```python
from build123d import *

# Parameters (mm, degrees)
F1_DEPTH = 50
F2_R     = 3.15
F3_DEPTH = 2.5
F4_R     = 3.15
F5_DEPTH = 1
F6_R     = 5


with BuildPart() as f1:
    # F0 (on Top) → F1 (new body)
    with BuildSketch(Plane.XY):
        with BuildLine():
            ThreePointArc((4.9458041958, 3.6553414145), (0, -6.15), (-4.9458041958, 3.6553414145))
            ThreePointArc((-4.9458041958, 3.6553414145), (-4.7531001977, 4.3283874081), (-5.0490024533, 4.9628695557))
            Line((-5.0490024533, 4.9628695557), (-5.7683657215, 5.669960926))
            ThreePointArc((-5.7683657215, 5.669960926), (-6.5394133994, 5.9543407148), (-7.2631501723, 5.5649932232))
            ThreePointArc((-7.2631501723, 5.5649932232), (-8.6851191985, -2.8794451737), (-2.5, -8.8018463972))
            Line((-2.5, -8.8018463972), (2.5, -8.8018463972))
            ThreePointArc((2.5, -8.8018463972), (8.6851191985, -2.8794451737), (7.2631501723, 5.5649932232))
            ThreePointArc((7.2631501723, 5.5649932232), (6.5394133994, 5.9543407148), (5.7683657215, 5.669960926))
            Line((5.7683657215, 5.669960926), (5.0490024533, 4.9628695557))
            ThreePointArc((5.0490024533, 4.9628695557), (4.7531001977, 4.3283874081), (4.9458041958, 3.6553414145))
        make_face()
    extrude(amount=F1_DEPTH)

    # F2 (on Right) → F3 (join, symmetric)
    with BuildSketch(Plane.YZ):
        with BuildLine():
            Line((-41.1023570115, 34.5058199478), (-8.8018463972, 0))
            Line((-8.8018463972, 0), (-8.8018463972, 50))
            Line((-8.8018463972, 50), (-38.8018463972, 50))
            ThreePointArc((-38.8018463972, 50), (-43.6934106929, 42.8084037793), (-41.1023570115, 34.5058199478))
        make_face()
        with Locations((-33.8018463972, 41.3397459622)):
            Circle(F2_R, mode=Mode.SUBTRACT)
    extrude(amount=F3_DEPTH, both=True)

    # F4 (on face) → F5 (cut)
    with BuildSketch(Plane(origin=(-2.5, 0, 0), x_dir=(0, -1, 0), z_dir=(-1, 0, 0))):
        Polygon((36.7752002835, 46.4897459622), (30.8284925109, 46.4897459622), (27.8551386246, 41.3397459622), (30.8284925109, 36.1897459622), (36.7752002835, 36.1897459622), (39.7485541699, 41.3397459622), align=None)
        with Locations((33.8018463972, 41.3397459622)):
            Circle(F4_R, mode=Mode.SUBTRACT)
    extrude(amount=-F5_DEPTH, mode=Mode.SUBTRACT)

    # F6 (call 1 of 2: OpenCascade refuses the feature's edges together)
    f6_edges = [f1.edges().sort_by_distance(p)[0] for p in [
        (2.5, -8.801846, 25),
    ]]
    fillet(f6_edges, radius=F6_R)

    # F6#2 (call 2 of 2)
    f6_2_edges = [f1.edges().sort_by_distance(p)[0] for p in [
        (-2.5, -8.801846, 25),
    ]]
    fillet(f6_2_edges, radius=F6_R)


solid = f1.part
```
Geometry check sheet. Reference: the model listing, model coordinates, mm. A direction names the side the tool comes from. Coordinates: 2 decimals unless noted, no trailing zeros. Write each loop counter-clockwise with the first axis right and the second up, starting at its lowest first coordinate (ties: lowest second). Pieces come first, ordered by that corner, then holes. Notation, with made-up numbers: M -16,6 L 23,6 A35 cw 23,43 Z; hole C -27.5,7 d2. An arc over 180 degrees is marked long. Answer as a JSON object with one key per item and string values.
1. Scan lines: L1, parallel to X at y = 0, z = 26.5; L2, parallel to Y at x = -2, z = 40.5; L3, parallel to Z at x = -1.75, y = -29. Record each from-to range of solid material in increasing order.
Answers below:
{"L1": "x = -9.15 to -6.15, 6.15 to 9.15", "L2": "y = -43.77 to -39.26, -28.34 to -5.82", "L3": "z = 21.58 to 39.36, 43.32 to 50"}
2. Section check D-D, the plane y = -32.5. Enter the section's corners in (x, z), plus the area to 3 significant figures.
Answers below:
{"outline": "M -2.5,25.32 L 2.5,25.32 L 2.5,38.47 L -1.5,38.47 L -1.5,36.19 L -2.5,36.19 Z; M -2.5,46.49 L -1.5,46.49 L -1.5,44.21 L 2.5,44.21 L 2.5,50 L -2.5,50 Z", "area": "90.2 mm²"}
3. Draft check along X on faces 1 (the cylindrical face through (4.754, 4.338, 24.65)), 2 (the cylindrical face through (-9.02, -1.53, 24.65)), 3 (the flat face through (0, -16, 50)). Enter one of: released by +X, released by -X, zero draft, split by the parting line, or undercut.
Answers below:
{"face 1": "undercut", "face 2": "released by -X", "face 3": "zero draft"}
4. Section check A-A, the plane y = 0. Enter the section's corners in (x, z), plus the area to 3 significant figures.
Answers below:
{"outline": "M -9.15,0 L -6.15,0 L -6.15,50 L -9.15,50 Z; M 6.15,0 L 9.15,0 L 9.15,50 L 6.15,50 Z", "area": "300 mm²"}
5. Section check C-C, the plane z = 23. Enter the section's corners in (x, y) (3 decimals), plus the area to 3 significant figures.
Answers below:
{"outline": "M -7.263,5.565 A9.15 ccw -4.85,-7.759 A5 cw -2.5,-11.999 L -2.5,-30.332 L 2.5,-30.332 L 2.5,-11.999 A5 cw 4.85,-7.759 A9.15 ccw 7.263,5.565 A1 ccw 5.768,5.67 L 5.049,4.963 A1 ccw 4.946,3.655 A6.15 cw long -4.946,3.655 A1 ccw -5.049,4.963 L -5.768,5.67 A1 ccw Z", "area": "216 mm²"}
6. Tool access check on faces 4 (the flat face through (2.5, -25, 32)), 5 (the flat face through (-2.01, -29.36, 43.95)), 6 (the cylindrical face through (-4.752, 4.318, 24.65)), 7 (the flat face through (-2.5, -25, 32)). Record the directions out of +Z, -Z, +X, -X, +Y, -Y that give a thin tool (end or side, any length) a straight path to the whole face; none if there is none.
Answers below:
{"face 4": "+Z, -Z, +X, -Y", "face 5": "-X", "face 6": "+Z, -Z", "face 7": "+Z, -Z, -X, -Y"}
7. Section check B-B, the plane x = 0. Enter the section's corners in (y, z).
Answers below:
{"outline": "M -41.1,34.51 L -8.8,0 L -6.15,0 L -6.15,50 L -38.8,50 A10 ccw Z; hole C -33.8,41.34 d6.3"}
8. Go/stop test with flat-tipped pins: pin 1 Ø2 at (x, z) = (6.5, 39.5) entering from -Y; pin 2 Ø5 at (y, z) = (-36, 42.5) entering from -X; pin 3 Ø9.5 at (y, z) = (-32.5, 21.5) entering from +X; pin 4 Ø9.5 at (y, z) = (-35, 18.5) entering from -X. Record where each tip stops, or that it passes through.
Answers below:
{"pin 1": "stops at y = -7.31", "pin 2": "stops at x = -1.5", "pin 3": "stops at x = 2.5", "pin 4": "passes through"}
